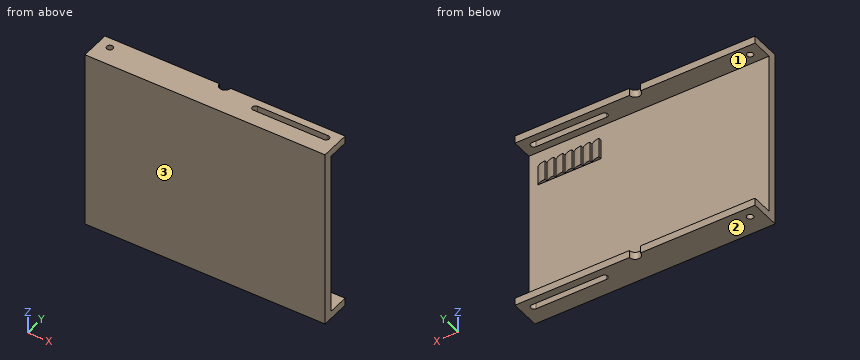
```python
from build123d import *

# Parameters (mm, degrees)
AUFSATZ_LINEAR_AUSTRAGEN3_DEPTH      = 80
SCHNITT_LINEAR_AUSTRAGEN1_DEPTH      = 146.602197786
SCHNITT_LINEAR_AUSTRAGEN1_DEPTH_BACK = 146.602197786
SKIZZE10_R                           = 2.1
SCHNITT_LINEAR_AUSTRAGEN2_DEPTH      = 102.980390272
SCHNITT_LINEAR_AUSTRAGEN2_DEPTH_BACK = 102.980390272
AUFSATZ_LINEAR_AUSTRAGEN4_DEPTH      = 45
LINEARES_MUSTER1_COUNT               = 7
LINEARES_MUSTER1_PITCH               = 6
SKIZZE19_W                           = 160
SKIZZE19_H                           = 14
SCHNITT_LINEAR_AUSTRAGEN3_DEPTH      = 32


with BuildPart() as part:
    # Skizze9 → Aufsatz-Linear austragen3 (new, symmetric)
    with BuildSketch(Plane(origin=(0, 0, 0), x_dir=(0, 0, -1), z_dir=(1, 0, 0))):
        Polygon((-60, 20), (-60, 0), (60, 0), (60, 20), (55, 20), (55, 6), (-55, 6), (-55, 20), align=None)
    extrude(amount=AUFSATZ_LINEAR_AUSTRAGEN3_DEPTH, both=True)

    # Skizze10 → Schnitt-Linear austragen1 (cut, two sides: drawn at the far end of the back side and taken through both)
    with BuildSketch(Plane.XY.offset(60).offset(-SCHNITT_LINEAR_AUSTRAGEN1_DEPTH_BACK)):
        with Locations((-72, 13)):
            Circle(SKIZZE10_R)
        with BuildLine():
            Line((25, 15.1), (72, 15.1))
            ThreePointArc((72, 15.1), (74.1, 13), (72, 10.9))
            Line((72, 10.9), (25, 10.9))
            ThreePointArc((25, 10.9), (22.9, 13), (25, 15.1))
        make_face()
    extrude(amount=SCHNITT_LINEAR_AUSTRAGEN1_DEPTH + SCHNITT_LINEAR_AUSTRAGEN1_DEPTH_BACK, mode=Mode.SUBTRACT)

    # Skizze12 → Schnitt-Linear austragen2 (cut, two sides: drawn at the far end of the back side and taken through both)
    with BuildSketch(Plane.XY.offset(-SCHNITT_LINEAR_AUSTRAGEN2_DEPTH_BACK)):
        with BuildLine():
            Line((-3.7, 20), (3.7, 20))
            ThreePointArc((3.7, 20), (0, 16.3), (-3.7, 20))
        make_face()
    extrude(amount=SCHNITT_LINEAR_AUSTRAGEN2_DEPTH + SCHNITT_LINEAR_AUSTRAGEN2_DEPTH_BACK, mode=Mode.SUBTRACT)

    # Skizze18 → Aufsatz-Linear austragen4 (add)
    with BuildSketch(Plane(origin=(0, 0, 0), x_dir=(-1, 0, 0), z_dir=(0, 0, -1))):
        with BuildLine():
            Line((-32, 6), (-38, 6))
            add(Edge.make_bspline(
                [(-38, 6), (-35.16767955, 8.124664511), (-32, 8)],
                knots=[0, 0, 0, 0.477297659, 0.477297659, 0.477297659], degree=2))
            Line((-32, 8), (-32, 6))
        make_face()
    aufsatz_linear_austragen4 = extrude(amount=-AUFSATZ_LINEAR_AUSTRAGEN4_DEPTH)

    # Lineares Muster1: Aufsatz-Linear austragen4 ×7
    with Locations(*[(i * LINEARES_MUSTER1_PITCH, 0, 0) for i in range(1, LINEARES_MUSTER1_COUNT)]):
        add(aufsatz_linear_austragen4)

    # Skizze19 → Schnitt-Linear austragen3 (cut)
    with BuildSketch(Plane.XY):
        with Locations((0, 13)):
            Rectangle(SKIZZE19_W, SKIZZE19_H)
    extrude(amount=SCHNITT_LINEAR_AUSTRAGEN3_DEPTH, mode=Mode.SUBTRACT)


solid = part.part
```
Source: CAD feature listing. Evaluate the final solid. Frame: model axes, mm. Face numbers are marked on the shaded views. Round coordinates to 2 decimals unless told otherwise and drop trailing zeros. Write each loop counter-clockwise with the first axis right and the second up, starting at its lowest first coordinate (ties: lowest second). Pieces come first, ordered by that corner, then holes. Notation, with made-up numbers: M -3.5,41 L 33.5,41 A24 ccw 33.5,65 Z; hole C -24.5,67.25 d2. An arc over 180 degrees is marked long. Answer as a JSON object with one key per item and string values. Group by question number.
(1) Section query B-B on x = -72. Output: boundary loops of the cut face in (y, z).
(2) Section query C-C on x = -50. Output: boundary loops of the cut face in (y, z).
(3) Mould query, pull axis Z, two halves, no side actions, for the marked faces 1, 2 and 3. Classes: +Z half, -Z half, draft (parallel to the pull), parting line (faces both ways), or undercut.
(4) Section query A-A on y = 13. Output: boundary loops of the cut face in (x, z), then the cut area to 3 significant figures.
(5) Ray query, line 1 (X direction, y = 13, z = 58.35); line 2 (Z direction, x = -23, y = 13.5); line 3 (Y direction, x = -72, z = 57.1). Return the intervals inside material, ascending. Write a range as [from, to].
(6) First-contact query: pin 1 (1.5 mm diameter, centred on x = -9.5, z = 22, fed in from +Y); pin 2 (1.6 mm diameter, centred on y = 7, z = 38, fed in from -X); pin 3 (4 mm diameter, centred on x = 40.5, z = 56.5, fed in from -Y). Flat tips, straight axial feed; report the tip coordinate or a pass-through.
(7) Section query D-D on z = -51.5. Output: boundary loops of the cut face in (x, y).
Computed values:
{
 "1": {"outline": "M 0,-60 L 10.9,-60 L 10.9,-55 L 6,-55 L 6,55 L 10.9,55 L 10.9,60 L 0,60 Z; M 15.1,-60 L 20,-60 L 20,-55 L 15.1,-55 Z; M 15.1,55 L 20,55 L 20,60 L 15.1,60 Z"},
 "2": {"outline": "M 0,-60 L 20,-60 L 20,-55 L 6,-55 L 6,55 L 20,55 L 20,60 L 0,60 Z"},
 "3": {"face 1": "undercut", "face 2": "-Z half", "face 3": "draft"},
 "4": {"outline": "M -80,-60 L -74.1,-60 L -74.1,-55 L -80,-55 Z; M -80,55 L -74.1,55 L -74.1,60 L -80,60 Z; M -69.9,-60 L 22.9,-60 L 22.9,-55 L -69.9,-55 Z; M -69.9,55 L 22.9,55 L 22.9,60 L -69.9,60 Z; M 74.1,-60 L 80,-60 L 80,-55 L 74.1,-55 Z; M 74.1,55 L 80,55 L 80,60 L 74.1,60 Z", "area": "1,050 mm^2"},
 "5": {"line 1": "[-80, -74.1], [-69.9, 22.9], [74.1, 80]", "line 2": "[-60, -55], [55, 60]", "line 3": "[0, 10.9], [15.1, 20]"},
 "6": {"pin 1": "y = 6", "pin 2": "x = 32", "pin 3": "y = 0"},
 "7": {"outline": "M -80,0 L 80,0 L 80,6 L -80,6 Z"}
}
